Geometry check sheet. Reference: the model listing, model coordinates, mm. Face numbers are marked on the shaded views. A direction names the side the tool comes from. Coordinates: 2 decimals unless noted, no trailing zeros. Order: outer loops, then holes, each group sorted by start corner. A loop starts at its lowest first (then second) coordinate and runs counter-clockwise, first axis right, second up. Notation, with made-up numbers: (59.25, -22) - (117.25, -22) arc R16 cw to (117.25, -11) - close; hole circle Ø5 at (19.25, 60). An arc over 180 degrees is marked (long way). Return JSON: item names as keys, results as strings. Group by question number.
Item 1: Section check B-B on y = -1. Enter the section's corners in (x, z), then the cut area to 3 significant figures.
Item 2: Draft check along X on the marked faces 3, 4 and 5. Enter one of: pulls with the +X half, pulls with the -X half, needs draft (parallel to the pull), parting line crosses it, or undercut.
Item 3: Tool access check on the marked faces 1 and 2. Record the directions out of +Z, -Z, +X, -X, +Y, -Y that give a thin tool (end or side, any length) a straight path to the whole face; none if there is none.
Item 4: Scan lines: probe 1 along X at (y, z) = (0.75, -6.5); probe 2 along Z at (x, y) = (-0.75, 0); probe 3 along X at (y, z) = (-2, -27). Record each from-to range of solid material in increasing order.
Item 5: Gauge pin test, flat ends, axial feed: pin 1 (1 mm diameter, centred on y = -2, z = -4.5, fed in from -X); pin 2 (3 mm diameter, centred on y = 2.5, z = -29, fed in from +X); pin 3 (4 mm diameter, centred on y = 1, z = -31.5, fed in from -X). Record the tip position at first contact, or that the pin passes through.
Item 6: Section check A-A on z = -23.5. Enter the section's corners in (x, y), then the cut area to 3 significant figures.
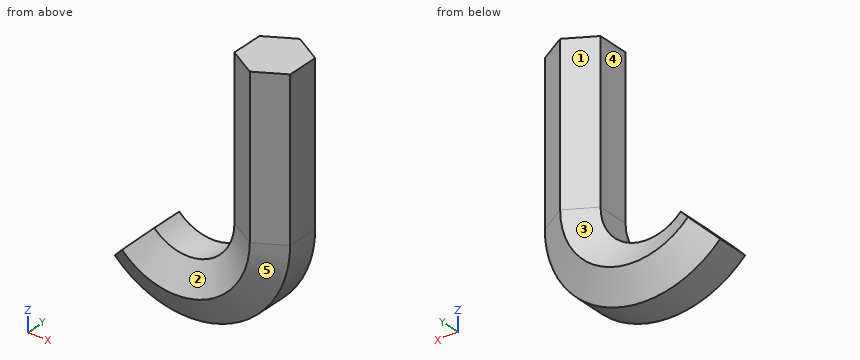
from build123d import *


with BuildPart() as f2:
    # F2: sweep along a path in F0
    with BuildLine(Plane.XZ) as f2_path:
        Line((0, 0), (0, -24.370959))
        ThreePointArc((0, -24.370959), (-7.179451, -35.115767), (-19.853817, -32.594679))
    # F1 (on Top) → F2 (sweep)
    with BuildSketch(Plane.XY):
        Polygon((-4.330127, -2.5), (0, -5), (4.330127, -2.5), (4.330127, 2.5), (0, 5), (-4.330127, 2.5), align=None)
    sweep(path=f2_path.line)


solid = f2.part
Computed:
{
 "1": {"outline": "(-22.92, -35.66) arc R15.96 ccw to (4.33, -24.37) - (4.33, 0) - (-4.33, 0) - (-4.33, -24.37) arc R7.3 cw to (-16.79, -29.53) - close", "area": "448 mm²"},
 "2": {"face 3": "undercut", "face 4": "pulls with the -X half", "face 5": "parting line crosses it"},
 "3": {"face 1": "+Z, -X, +Y", "face 2": "+Z, -Y"},
 "4": {"probe 1": "x = -4.33 to 4.33", "probe 2": "z = -36.05 to 0", "probe 3": "x = -4.82 to 4.11"},
 "5": {"pin 1": "stops at x = -4.33", "pin 2": "stops at x = 4.02", "pin 3": "stops at x = -20.76"},
 "6": {"outline": "(-4.33, -2.5) - (0, -5) - (4.33, -2.5) - (4.33, 2.5) - (0, 5) - (-4.33, 2.5) - close", "area": "65.0 mm²"}
}
